Source: CAD feature listing. Evaluate the final solid. Frame: model axes, mm. A direction names the side the tool comes from. Give positions to 0.01 mm unless a question says otherwise; leave off trailing zeros. Order: outer loops, then holes, each group sorted by start corner. A loop starts at its lowest first (then second) coordinate and runs counter-clockwise, first axis right, second up. Notation, with made-up numbers: (55, 1) - (70, 1) arc R20 cw to (70, 27) - close; hole circle Ø6 at (52, 37). An arc over 180 degrees is marked (long way). Use CSV: the item, a comma, the result in double quotes.
```python
from build123d import *

# Parameters (mm, degrees)
GUIDE_AND_SOLID_STOPS_DEPTH   = 13.6
SKETCH_3_W                    = 8.4
SKETCH_3_H                    = 14
NUT_TONGUE_CHANNEL_DEPTH      = 2.8
SKETCH_4_W                    = 6.25
SKETCH_4_H                    = 5.2
LOWER_YOKE_RELIEF_DEPTH       = 3
SKETCH_5_W                    = 3.7
SKETCH_5_H                    = 3
LOWER_INWARD_STOP_DEPTH       = 3.8
SKETCH_7_W                    = 3.7
SKETCH_7_H                    = 3
EXTRUDE_2_DEPTH               = 3.8
REMOVE_LOWER_TAIL_DEPTH       = 62.002151601
REMOVE_LOWER_TAIL_DEPTH_BACK  = 62.002151601
SKETCH_8_W                    = 17
SKETCH_8_H                    = 17
WIDER_SHAFT_RELIEF_DEPTH      = 62.002151601
WIDER_SHAFT_RELIEF_DEPTH_BACK = 62.002151601
SKETCH_9_W                    = 9.85
SKETCH_9_H                    = 46


with BuildPart() as part:
    # 草图1 → Guide_and_solid_stops (new body)
    with BuildSketch(Plane.XY):
        Polygon((-10.2, 0), (-16.95, 0), (-16.95, 54), (-11.2, 54), (-11.2, 57), (-4.7, 57), (-4.7, 53), (-10.2, 53), (-10.2, 51.5), (-10.95, 51.5), (-10.95, 38), (-10.2, 38), (-10.2, 36), (-4.7, 36), (-4.7, 32), (-10.2, 32), align=None)
    extrude(amount=GUIDE_AND_SOLID_STOPS_DEPTH)

    # 草图3 → Nut_tongue_channel (cut, symmetric)
    with BuildSketch(Plane.XY.offset(6.8)):
        with Locations((-11.2, 44.5)):
            Rectangle(SKETCH_3_W, SKETCH_3_H)
    extrude(amount=NUT_TONGUE_CHANNEL_DEPTH, both=True, mode=Mode.SUBTRACT)

    # 草图4 → Lower_yoke_relief (cut, symmetric)
    with BuildSketch(Plane.XY.offset(6.8)):
        with Locations((-7.125, 33.6)):
            Rectangle(SKETCH_4_W, SKETCH_4_H)
    extrude(amount=LOWER_YOKE_RELIEF_DEPTH, both=True, mode=Mode.SUBTRACT)

    # 草图5 → Lower_inward_stop (add)
    with BuildSketch(Plane.XY):
        with Locations((-9.35, 16.5)):
            Rectangle(SKETCH_5_W, SKETCH_5_H)
    extrude(amount=LOWER_INWARD_STOP_DEPTH)

    # 草图7 → 凸台-拉伸2 (add)
    with BuildSketch(Plane.XY.offset(9.8)):
        with Locations((-9.35, 16.5)):
            Rectangle(SKETCH_7_W, SKETCH_7_H)
    extrude(amount=EXTRUDE_2_DEPTH)

    # 草图8 → Remove_lower_tail (cut, two sides: drawn at the far end of the back side and taken through both)
    with BuildSketch(Plane.XY.offset(-REMOVE_LOWER_TAIL_DEPTH_BACK)):
        with Locations((-11.5, 6.5)):
            Rectangle(SKETCH_8_W, SKETCH_8_H)
    extrude(amount=REMOVE_LOWER_TAIL_DEPTH + REMOVE_LOWER_TAIL_DEPTH_BACK, mode=Mode.SUBTRACT)

    # 草图9 → Wider_shaft_relief (cut, two sides: drawn at the far end of the back side and taken through both)
    with BuildSketch(Plane.XY.offset(-WIDER_SHAFT_RELIEF_DEPTH_BACK)):
        with Locations((-4.925, 36)):
            Rectangle(SKETCH_9_W, SKETCH_9_H)
    extrude(amount=WIDER_SHAFT_RELIEF_DEPTH + WIDER_SHAFT_RELIEF_DEPTH_BACK, mode=Mode.SUBTRACT)


solid = part.part
```
Item 1: Section B-B on x = -12.25. Return the cut outline in (y, z), then the cut area to 3 significant figures.
Filled in:
outline,"(15, 0) - (54, 0) - (54, 13.6) - (15, 13.6) - close; hole (37.5, 4) - (51.5, 4) - (51.5, 9.6) - (37.5, 9.6) - close"
area,"452 mm2"
Item 2: Section C-C on z = 7. Return the cut outline in (x, y), then the cut area to 3 significant figures.
Filled in:
outline,"(-16.95, 15) - (-10.2, 15) - (-10.2, 31) - (-10.25, 31) - (-10.25, 36.2) - (-10.2, 36.2) - (-10.2, 37.5) - (-15.4, 37.5) - (-15.4, 51.5) - (-10.2, 51.5) - (-10.2, 53) - (-9.85, 53) - (-9.85, 57) - (-11.2, 57) - (-11.2, 54) - (-16.95, 54) - close"
area,"195 mm2"
Item 3: Section D-D on y = 35.5. Return the cut outline in (x, z).
Filled in:
outline,"(-16.95, 0) - (-9.85, 0) - (-9.85, 3.8) - (-10.25, 3.8) - (-10.25, 9.8) - (-9.85, 9.8) - (-9.85, 13.6) - (-16.95, 13.6) - close"
Item 4: Set-up query: faces 4 (the flat face through (-10.2, 37, 7)), 5 (the flat face through (-10.25, 34, 7)), 6 (the flat face through (-14, 54, 7)). Return all of +Z, -Z, +X, -X, +Y, -Y with unobstructed straight access to the full face (end or side cutting, diameter ignored); none if empty.
Filled in:
face 4,"+Z, -Z, +X"
face 5,"+X"
face 6,"+Z, -Z, -X, +Y"
Item 5: Mould query, pull axis Z, two halves, no side actions, for faces 1 (the flat face through (-9.85, 16, 2)), 2 (the flat face through (-13, 37.5, 7)), 3 (the flat face through (-13, 36, 13.6)). Classes: released by +Z, released by -Z, zero draft, split by the parting line, or undercut.
Filled in:
face 1,"zero draft"
face 2,"undercut"
face 3,"released by +Z"
Item 6: First-contact query: pin 1 (1 mm diameter, centred on x = -16, z = 4, fed in from +Y); pin 2 (2 mm diameter, centred on x = -14.5, y = 48, fed in from -Z); pin 3 (1 mm diameter, centred on y = 20, z = 7.5, fed in from +X); pin 4 (4.5 mm diameter, centred on y = 47.5, z = 12, fed in from +X). Flat tips, straight axial feed; report the tip coordinate or a pass-through.
Filled in:
pin 1,"stops at y = 54"
pin 2,"stops at z = 0"
pin 3,"stops at x = -10.2"
pin 4,"stops at x = -10.95"
Item 7: Section A-A on y = 49. Return the cut outline in (x, z), then the cut area to 3 significant figures.
Filled in:
outline,"(-16.95, 0) - (-10.95, 0) - (-10.95, 4) - (-15.4, 4) - (-15.4, 9.6) - (-10.95, 9.6) - (-10.95, 13.6) - (-16.95, 13.6) - close"
area,"56.7 mm2"
Item 8: Material intervals for line 1 (Y direction, x = -14, z = 5.5); line 2 (Y direction, x = -10.5, z = 8.25); line 3 (Z direction, x = -14, y = 41), sorted ascending. Write a range as from..to.
Filled in:
line 1,"y = 15..37.5, 51.5..54"
line 2,"y = 15..37.5, 51.5..57"
line 3,"z = 0..4, 9.6..13.6"
